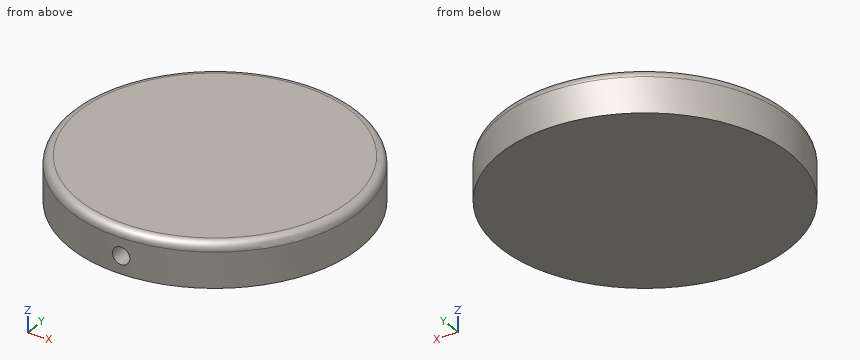
```python
from build123d import *

# Parameters (mm, degrees)
F0_R     = 166.5
F1_DEPTH = 50.8
F2_R     = 10
F4_R     = 10
F5_DEPTH = 97.282


with BuildPart() as f1:
    # F0 (on Top) → F1 (new body)
    with BuildSketch(Plane.XY):
        Circle(F0_R)
    extrude(amount=F1_DEPTH)

    # F2
    f2_edges = [f1.edges().sort_by_distance(p)[0] for p in [
        (-166.5, 0, 50.8),
    ]]
    fillet(f2_edges, radius=F2_R)

    # F4 (on offset) → F5 (cut)
    with BuildSketch(Plane.XZ.offset(167.132)):
        with Locations((0, 20.608293)):
            Circle(F4_R)
    extrude(amount=-F5_DEPTH, mode=Mode.SUBTRACT)


solid = f1.part
```
The listing builds one solid part. Answer for the finished solid, in the listing's coordinates (mm). Coordinates: 2 decimals unless noted, no trailing zeros. Write each loop counter-clockwise with the first axis right and the second up, starting at its lowest first coordinate (ties: lowest second). Pieces come first, ordered by that corner, then holes.
Q1. Section A-A, the plane x = 0 is taken. Write down the section's boundary in (y, z).
Returned:
outline: (-166.5, 0) - (166.5, 0) - (166.5, 40.8) arc R10 ccw to (156.5, 50.8) - (-156.5, 50.8) arc R10 ccw to (-166.5, 40.8) - (-166.5, 30.61) - (-69.85, 30.61) - (-69.85, 10.61) - (-166.5, 10.61) - close
Q2. Given P1, Ø5, axis at y = -21, z = 36.5, coming from the -X side; P2, Ø8, axis at x = -81.5, z = 20, coming from the +Y side; P3, Ø2, axis at x = 7.5, z = 23, coming from the +Y side, each flat-ended and moving along its own axis, determine where each tip first touches the part or whether it passes through.
Returned:
P1: stops at x = -165.47
P2: stops at y = 147.36
P3: stops at y = 166.37
Q3. Find the intervals of material crossed by line 1 along Z through (x, y) = (0, -102.5); line 2 along Y through (x, z) = (54, 45); line 3 along Y through (x, z) = (-3.5, 10), in increasing order.
Returned:
line 1: z = 0 to 10.61, 30.61 to 50.8
line 2: y = -156.52 to 156.52
line 3: y = -166.46 to 166.46
Q4. Section B-B, the plane z = 34.5 is taken. Write down the section's boundary in (x, y).
Returned:
outline: circle Ø333 at (0, 0)
